Work out the finished part from the listing and answer in its coordinate system (mm). A direction names the side the tool comes from. Give positions to 0.01 mm unless a question says otherwise; leave off trailing zeros. Loops run counter-clockwise (first coordinate to the right, second up) from the corner with the lowest first, then second, coordinate; pieces in that order, holes last.
from build123d import *

# Parameters (mm, degrees)
F1_DEPTH = 10
F3_D     = 0.5
F5_D     = 0.5
F8_DEPTH = 5
F9_R     = 0.5
F10_R    = 0.5
F11_R    = 0.5


with BuildPart() as f1:
    # F0 (on Front) → F1 (new body)
    with BuildSketch(Plane.XZ):
        Polygon((-10, 0), (0, 0), (0, 1), (-1, 1), (-2, 1), (-10, 1), align=None)
        with BuildLine():
            Line((-1, 1), (0, 1))
            Line((0, 1), (0, 2))
            ThreePointArc((0, 2), (-0.2928932188, 1.2928932188), (-1, 1))
        make_face()
        with BuildLine():
            Line((-2, 1), (-1, 1))
            ThreePointArc((-1, 1), (-1.7071067812, 1.2928932188), (-2, 2))
            Line((-2, 2), (-2, 1))
        make_face()
        with BuildLine():
            ThreePointArc((-2, 2), (-1.7071067812, 1.2928932188), (-1, 1))
            ThreePointArc((-1, 1), (-0.2928932188, 1.2928932188), (0, 2))
            ThreePointArc((0, 2), (-1, 3), (-2, 2))
        make_face()
    extrude(amount=F1_DEPTH)

    # F3 (through all)
    with Locations(Plane.XY.offset(1)):
        with Locations((-8, -2), (-8.8854947245, -8), (-4, -8), (-4, -2)):
            Hole(F3_D / 2)

    # F5 (through all)
    with Locations(Plane.XZ.offset(10)):
        with Locations((-1, 2)):
            Hole(F5_D / 2)

    # F7 (on offset) → F8 (cut)
    with BuildSketch(Plane.XZ.offset(7.5)):
        with BuildLine():
            ThreePointArc((-2, 2), (-1, 1), (0, 2))
            ThreePointArc((0, 2), (-1, 3), (-2, 2))
        make_face()
        with BuildLine():
            Line((0, 0), (0, 2))
            ThreePointArc((0, 2), (-1, 1), (-2, 2))
            Line((-2, 2), (-2, 1))
            Line((-2, 1), (0, 0))
        make_face()
    extrude(amount=-F8_DEPTH, mode=Mode.SUBTRACT)

    # F9
    f9_edges = [f1.edges().sort_by_distance(p)[0] for p in [
        (-10, -5, 1),
        (-6, -10, 1),
        (-6, 0, 1),
    ]]
    fillet(f9_edges, radius=F9_R)

    # F10
    f10_edges = [f1.edges().sort_by_distance(p)[0] for p in [
        (0, -10, 1),
        (-1, -10, 3),
        (-2, -10, 1.5),
    ]]
    fillet(f10_edges, radius=F10_R)

    # F11
    f11_edges = [f1.edges().sort_by_distance(p)[0] for p in [
        (-2, 0, 1.5),
        (0, 0, 1),
        (-1, 0, 3),
    ]]
    fillet(f11_edges, radius=F11_R)


solid = f1.part
Item 1: Find section B-B, the plane z = 0.35. Write down the section's boundary in (x, y).
Item 2: Consider line 1 (Y direction, x = -4, z = 0.45); line 2 (Z direction, x = -1, y = -0.65); line 3 (Y direction, x = -8, z = 0.45). Determine where each line is inside the solid, lowest interval first.
Item 3: Find section D-D, the plane x = -6. Write down the section's boundary in (y, z), plus the area to 3 significant figures.
Item 4: Flat-ended cylindrical pins translate along their axes: pin 1 Ø4 at (x, y) = (-7.5, -7) entering from +Z; pin 2 Ø0.5 at (y, z) = (-2, 1.5) entering from -X; pin 3 Ø1 at (x, z) = (-8, 2.5) entering from -Y. Find the tip coordinate at first contact, or state that the pin passes through.
Item 5: Find section A-A, the plane x = -4. Write down the section's boundary in (y, z), plus the area to 3 significant figures.
Item 6: For faces 1 (the face through (-1, -1, 3)), 2 (the face through (-1, -5, 0.5)), 3 (the face through (-2, -1.5, 1.5)), determine the directions among +Z, -Z, +X, -X, +Y, -Y from which every point of the face is accessible in a straight line to the end or side of a thin tool.
Item 7: Find section C-C, the plane x = -8. Write down the section's boundary in (y, z).
Ans:
1. outline: (-10, -10) - (-0.5, -10) arc R0.5 ccw to (0, -9.5) - (0, -7.5) - (-0.7, -7.5) - (-0.7, -2.5) - (0, -2.5) - (0, -0.5) arc R0.5 ccw to (-0.5, 0) - (-10, 0) - close; hole circle Ø0.5 at (-8.89, -8); hole circle Ø0.5 at (-8, -2); hole circle Ø0.5 at (-4, -8); hole circle Ø0.5 at (-4, -2)
2. line 1: y = -10 to -8.25, -7.75 to -2.25, -1.75 to 0
2. line 2: z = 0 to 1.75, 2.25 to 3
2. line 3: y = -10 to -2.25, -1.75 to 0
3. outline: (-10, 0) - (0, 0) - (0, 0.5) arc R0.5 ccw to (-0.5, 1) - (-9.5, 1) arc R0.5 ccw to (-10, 0.5) - close
3. area: 9.89 mm2
4. pin 1: stops at z = 1
4. pin 2: stops at x = -2
4. pin 3: passes through
5. outline: (-10, 0) - (-8.25, 0) - (-8.25, 1) - (-9.5, 1) arc R0.5 ccw to (-10, 0.5) - close; (-7.75, 0) - (-2.25, 0) - (-2.25, 1) - (-7.75, 1) - close; (-1.75, 0) - (0, 0) - (0, 0.5) arc R0.5 ccw to (-0.5, 1) - (-1.75, 1) - close
5. area: 8.89 mm2
6. face 1: +Z, +Y, -Y
6. face 2: +Z, +X
6. face 3: +Z, -X, +Y, -Y
7. outline: (-10, 0) - (-2.25, 0) - (-2.25, 1) - (-9.5, 1) arc R0.5 ccw to (-10, 0.5) - close; (-1.75, 0) - (0, 0) - (0, 0.5) arc R0.5 ccw to (-0.5, 1) - (-1.75, 1) - close
